Geometry: final body of the model. Coordinates: model frame, mm. A direction names the side the tool comes from. Round coordinates to 2 decimals unless told otherwise and drop trailing zeros. Loops run counter-clockwise (first coordinate to the right, second up) from the corner with the lowest first, then second, coordinate; pieces in that order, holes last. Notation, with made-up numbers: (-2, 8) - (17, 8) arc R18 ccw to (17, 23) - close; hole circle Ø3 at (-24, -29.75). An arc over 180 degrees is marked (long way). Return JSON: item names as keys, results as strings. Group by question number.
1. Material intervals for probe 1 along X at (y, z) = (-1.55, -31); probe 2 along X at (y, z) = (-8.5, -48); probe 3 along Z at (x, y) = (30, -9), sorted ascending.
2. Section B-B on z = -31. Return loops of the section in (x, y), and give its area (3 significant figures).
3. Set-up query: faces 4 (the face through (88, -8, -86)), 5 (the face through (33.5, -1, -43)), 6 (the face through (88.797, -7.605, -88.859)). Return all of +Z, -Z, +X, -X, +Y, -Y with unobstructed straight access to the full face (end or side cutting, diameter ignored); none if empty.
4. First-contact query: pin 1 Ø4 at (x, z) = (28.27, -31) entering from +Y; pin 2 Ø4 at (x, z) = (77, -56.5) entering from -Y. Flat tips, straight axial feed; report the tip coordinate or a pass-through.
5. Section A-A on x = 14.27. Return loops of the section in (y, z), and give its area (3 significant figures).
6. Draft query along Z for faces 1 (the face through (75, -1, -72)), 2 (the face through (44, -7, -90)), 3 (the face through (1, -15, -42)). Return one class per face: +Z half, -Z half, draft (parallel to the pull), parting line (faces both ways), or undercut.
7. Section D-D on z = -70. Return loops of the section in (x, y), and give its area (3 significant figures).
8. Section C-C on x = 28.27. Return loops of the section in (y, z), and give its area (3 significant figures).
from build123d import *

# Parameters (mm, degrees)
SKETCH1_W           = 90
SKETCH1_H           = 90
BOSS_EXTRUDE1_DEPTH = 15
SKETCH2_W           = 24
SKETCH2_H           = 15
CUT_EXTRUDE1_DEPTH  = 15
SHELL1_T            = -2
SKETCH3_R           = 3.5
CUT_EXTRUDE2_DEPTH  = 4
SKETCH4_W           = 10
SKETCH4_H           = 10
CUT_EXTRUDE3_DEPTH  = 4
FILLET1_R           = 4


with BuildPart() as part:
    # Sketch1 → Boss-Extrude1 (new body)
    with BuildSketch(Plane(origin=(0, 0, 0), x_dir=(1, 0, 0), z_dir=(0, 1, 0))):
        with Locations((45, 45)):
            Rectangle(SKETCH1_W, SKETCH1_H)
    extrude(amount=-BOSS_EXTRUDE1_DEPTH)

    # Sketch2 → Cut-Extrude1 (cut)
    with BuildSketch(Plane(origin=(90, 0, 0), x_dir=(0, 0, -1), z_dir=(1, 0, 0))):
        with Locations((72, -7.5)):
            Rectangle(SKETCH2_W, SKETCH2_H)
    extrude(amount=-CUT_EXTRUDE1_DEPTH, mode=Mode.SUBTRACT)

    # Shell1
    shell1_openings = [part.faces().sort_by_distance(p)[0] for p in [
        (43.255813953, -15, -43.744186047),
        (82.5, -7.5, -60),
        (82.5, -7.5, -84),
        (75, -7.5, -72),
    ]]
    offset(amount=SHELL1_T, openings=shell1_openings, kind=Kind.INTERSECTION)

    # Sketch3 → Cut-Extrude2 (cut)
    with BuildSketch(Plane(origin=(0, 0, 0), x_dir=(1, 0, 0), z_dir=(0, 1, 0))):
        with Locations(Location((14.27, 31, 0), (0, 0, 270))):
            Circle(SKETCH3_R)
        with Locations(Location((28.27, 31, 0), (0, 0, 270))):
            Circle(SKETCH3_R)
        with Locations(Location((76.27, 31, 0), (0, 0, 270))):
            Circle(SKETCH3_R)
    extrude(amount=-CUT_EXTRUDE2_DEPTH, mode=Mode.SUBTRACT)

    # Sketch4 → Cut-Extrude3 (cut)
    with BuildSketch(Plane(origin=(0, 0, 0), x_dir=(1, 0, 0), z_dir=(0, 1, 0))):
        with Locations((14.53, 42.78)):
            Rectangle(SKETCH4_W, SKETCH4_H)
        with Locations((28.5, 42.78)):
            Rectangle(SKETCH4_W, SKETCH4_H)
        with Locations((16.43, 73.77)):
            Rectangle(SKETCH4_W, SKETCH4_H)
    extrude(amount=-CUT_EXTRUDE3_DEPTH, mode=Mode.SUBTRACT)

    # Fillet1
    fillet1_edges = [part.edges().sort_by_distance(p)[0] for p in [
        (0, -7.5, -90),
        (90, -7.5, -90),
        (90, -7.5, 0),
        (0, -7.5, 0),
    ]]
    fillet(fillet1_edges, radius=FILLET1_R)


solid = part.part
Taken from the geometry:
{
 "1": {"probe 1": "0 to 10.77, 17.77 to 24.77, 31.77 to 72.77, 79.77 to 90", "probe 2": "0 to 2, 88 to 90", "probe 3": "-90 to -88, -2 to 0"},
 "2": {"outline": "(0, -15) - (2, -15) - (2, -2) - (10.77, -2) - (10.77, 0) - (0, 0) - close; (17.77, -2) - (24.77, -2) - (24.77, 0) - (17.77, 0) - close; (31.77, -2) - (72.77, -2) - (72.77, 0) - (31.77, 0) - close; (79.77, -2) - (88, -2) - (88, -15) - (90, -15) - (90, 0) - (79.77, 0) - close", "area": "190 mm2"},
 "3": {"face 4": "-Y", "face 5": "+Y, -Y", "face 6": "-Z, +X, +Y, -Y"},
 "4": {"pin 1": "through", "pin 2": "y = -2"},
 "5": {"outline": "(-15, -90) - (0, -90) - (0, -78.77) - (-2, -78.77) - (-2, -88) - (-15, -88) - close; (-15, -2) - (-2, -2) - (-2, -27.5) - (0, -27.5) - (0, 0) - (-15, 0) - close; (-2, -68.77) - (0, -68.77) - (0, -47.78) - (-2, -47.78) - close; (-2, -37.78) - (0, -37.78) - (0, -34.5) - (-2, -34.5) - close", "area": "178 mm2"},
 "6": {"face 1": "undercut", "face 2": "-Z half", "face 3": "draft"},
 "7": {"outline": "(0, -15) - (2, -15) - (2, -2) - (11.43, -2) - (11.43, 0) - (0, 0) - close; (21.43, -2) - (75, -2) - (75, 0) - (21.43, 0) - close", "area": "156 mm2"},
 "8": {"outline": "(-15, -90) - (0, -90) - (0, -47.78) - (-2, -47.78) - (-2, -88) - (-15, -88) - close; (-15, -2) - (-2, -2) - (-2, -27.5) - (0, -27.5) - (0, 0) - (-15, 0) - close; (-2, -37.78) - (0, -37.78) - (0, -34.5) - (-2, -34.5) - close", "area": "198 mm2"}
}
